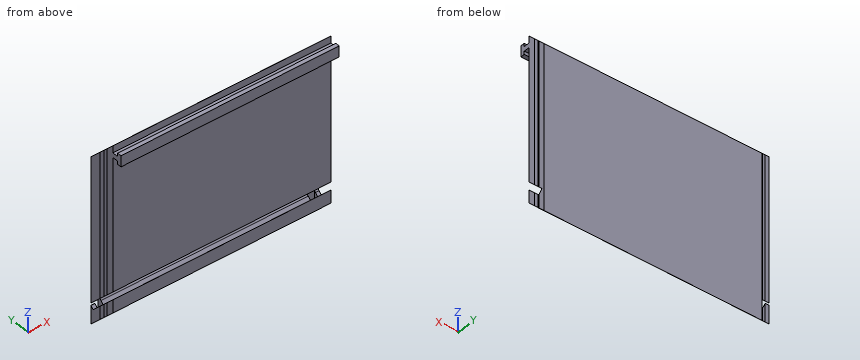
from build123d import *

# Parameters (mm, degrees)
SKETCH1_W           = 120
SKETCH1_H           = 100
BOSS_EXTRUDE1_DEPTH = 10
SKETCH2_W           = 6
SKETCH2_H           = 3
CUT_EXTRUDE1_DEPTH  = 120
SKETCH3_W           = 3
SKETCH3_H           = 1.75
CUT_EXTRUDE2_DEPTH  = 120
SKETCH4_W           = 3
SKETCH4_H           = 1.75
CUT_EXTRUDE3_DEPTH  = 120
SKETCH5_W           = 100
SKETCH5_H           = 3
BOSS_EXTRUDE2_DEPTH = 6
SKETCH6_W           = 3
SKETCH6_H           = 100
BOSS_EXTRUDE3_DEPTH = 1.75
SKETCH8_W           = 3
SKETCH8_H           = 100
BOSS_EXTRUDE4_DEPTH = 1.75
CUT_EXTRUDE4_DEPTH  = 140
CUT_EXTRUDE5_DEPTH  = 140
SKETCH12_W          = 120
SKETCH12_H          = 3
BOSS_EXTRUDE5_DEPTH = 6
SKETCH13_W          = 120
SKETCH13_H          = 3
BOSS_EXTRUDE6_DEPTH = 1.75
SKETCH14_W          = 120
SKETCH14_H          = 3
BOSS_EXTRUDE7_DEPTH = 1.75
SKETCH15_W          = 3.971349668
SKETCH15_H          = 100.27962334
CUT_EXTRUDE7_DEPTH  = 0.25
SKETCH16_W          = 3.977727367
SKETCH16_H          = 100.113606744
CUT_EXTRUDE8_DEPTH  = 0.25
SKETCH18_W          = 99.392543401
SKETCH18_H          = 7.459446395
CUT_EXTRUDE9_DEPTH  = 0.25
SKETCH19_W          = 3
SKETCH19_H          = 91.258373497
CUT_EXTRUDE10_DEPTH = 0.25
SKETCH22_W          = 3
SKETCH22_H          = 105.56058455
CUT_EXTRUDE11_DEPTH = 0.25
SKETCH23_W          = 145.417072626
SKETCH23_H          = 16.376201687
CUT_EXTRUDE12_DEPTH = 0.25
SKETCH24_W          = 92.054908244
SKETCH24_H          = 1.75
CUT_EXTRUDE13_DEPTH = 0.25
SKETCH25_W          = 91.75
SKETCH25_H          = 1.75
CUT_EXTRUDE14_DEPTH = 0.25
SKETCH27_W          = 146.123968395
SKETCH27_H          = 10.969132505
CUT_EXTRUDE15_DEPTH = 0.25
SKETCH28_W          = 131.910387722
SKETCH28_H          = 9.70209764
CUT_EXTRUDE16_DEPTH = 0.25
SKETCH29_W          = 147.06215687
SKETCH29_H          = 25.738379838
CUT_EXTRUDE17_DEPTH = 0.25
SKETCH30_W          = 120
SKETCH30_H          = 3
CUT_EXTRUDE18_DEPTH = 0.25
SKETCH31_W          = 120
SKETCH31_H          = 3
CUT_EXTRUDE19_DEPTH = 0.25
SKETCH32_W          = 120
SKETCH32_H          = 1.75
CUT_EXTRUDE20_DEPTH = 0.25
SKETCH33_W          = 120
SKETCH33_H          = 1.75
CUT_EXTRUDE21_DEPTH = 0.25
SKETCH36_W          = 96.5
SKETCH36_H          = 6.5
CUT_EXTRUDE23_DEPTH = 0.5
SKETCH39_W          = 96.5
SKETCH39_H          = 6.5
CUT_EXTRUDE27_DEPTH = 0.5
SKETCH41_W          = 4
SKETCH41_H          = 91.70363903
CUT_EXTRUDE28_DEPTH = 0.3
SKETCH42_W          = 3.987472746
SKETCH42_H          = 92.170181705
CUT_EXTRUDE29_DEPTH = 0.3
CUT_EXTRUDE30_DEPTH = 150
SKETCH44_W          = 120
SKETCH44_H          = 6
CUT_EXTRUDE31_DEPTH = 0.25
CUT_EXTRUDE32_DEPTH = 150


with BuildPart() as part:
    # Sketch1 → Boss-Extrude1 (new body)
    with BuildSketch(Plane(origin=(0, 0, 0), x_dir=(1, 0, 0), z_dir=(0, 1, 0))):
        with Locations((-60, -57.341499956)):
            Rectangle(SKETCH1_W, SKETCH1_H)
    extrude(amount=BOSS_EXTRUDE1_DEPTH)

    # Sketch2 → Cut-Extrude1 (cut)
    with BuildSketch(Plane(origin=(0, 0, 7.341499956), x_dir=(-1, 0, 0), z_dir=(0, 0, -1))):
        with Locations((3, 5)):
            Rectangle(SKETCH2_W, SKETCH2_H)
    extrude(amount=-CUT_EXTRUDE1_DEPTH, mode=Mode.SUBTRACT)

    # Sketch3 → Cut-Extrude2 (cut)
    with BuildSketch(Plane(origin=(0, 0, 7.341499956), x_dir=(-1, 0, 0), z_dir=(0, 0, -1))):
        with Locations((4.5, 7.375)):
            Rectangle(SKETCH3_W, SKETCH3_H)
    extrude(amount=-CUT_EXTRUDE2_DEPTH, mode=Mode.SUBTRACT)

    # Sketch4 → Cut-Extrude3 (cut)
    with BuildSketch(Plane(origin=(0, 0, 7.341499956), x_dir=(-1, 0, 0), z_dir=(0, 0, -1))):
        with Locations((4.5, 2.625)):
            Rectangle(SKETCH4_W, SKETCH4_H)
    extrude(amount=-CUT_EXTRUDE3_DEPTH, mode=Mode.SUBTRACT)

    # Sketch5 → Boss-Extrude2 (add)
    with BuildSketch(Plane.ZY.offset(120)):
        with Locations((57.341499956, 5)):
            Rectangle(SKETCH5_W, SKETCH5_H)
    extrude(amount=BOSS_EXTRUDE2_DEPTH)

    # Sketch6 → Boss-Extrude3 (add)
    with BuildSketch(Plane(origin=(0, 3.5, 0), x_dir=(-1, 0, 0), z_dir=(0, -1, 0))):
        with Locations((124.5, -57.341499956)):
            Rectangle(SKETCH6_W, SKETCH6_H)
    extrude(amount=BOSS_EXTRUDE3_DEPTH)

    # Sketch8 → Boss-Extrude4 (add)
    with BuildSketch(Plane(origin=(0, 6.5, 0), x_dir=(1, 0, 0), z_dir=(0, 1, 0))):
        with Locations((-124.5, -57.341499956)):
            Rectangle(SKETCH8_W, SKETCH8_H)
    extrude(amount=BOSS_EXTRUDE4_DEPTH)

    # Sketch9 → Cut-Extrude4 (cut)
    with BuildSketch(Plane(origin=(0, 0, 0), x_dir=(0, 0, -1), z_dir=(1, 0, 0))):
        Polygon((-7.341499956, 0), (-7.341499956, 10), (-17.341499956, 0), align=None)
    extrude(amount=-CUT_EXTRUDE4_DEPTH, mode=Mode.SUBTRACT)

    # Sketch10 → Cut-Extrude5 (cut)
    with BuildSketch(Plane(origin=(0, 0, 0), x_dir=(0, 0, -1), z_dir=(1, 0, 0))):
        Polygon((-107.341499956, 10), (-107.341499956, 0), (-97.341499956, 10), align=None)
    extrude(amount=-CUT_EXTRUDE5_DEPTH, mode=Mode.SUBTRACT)

    # Sketch12 → Boss-Extrude5 (add)
    with BuildSketch(Plane(origin=(0, 0, 0), x_dir=(-1, 0, 0), z_dir=(0, -1, 0))):
        with Locations((60, -102.341499956)):
            Rectangle(SKETCH12_W, SKETCH12_H)
    extrude(amount=BOSS_EXTRUDE5_DEPTH)

    # Sketch13 → Boss-Extrude6 (add)
    with BuildSketch(Plane(origin=(0, 0, 100.841499956), x_dir=(-1, 0, 0), z_dir=(0, 0, -1))):
        with Locations((60, -4.5)):
            Rectangle(SKETCH13_W, SKETCH13_H)
    extrude(amount=BOSS_EXTRUDE6_DEPTH)

    # Sketch14 → Boss-Extrude7 (add)
    with BuildSketch(Plane.XY.offset(103.841499956)):
        with Locations((-60, -4.5)):
            Rectangle(SKETCH14_W, SKETCH14_H)
    extrude(amount=BOSS_EXTRUDE7_DEPTH)

    # Sketch15 → Cut-Extrude7 (cut)
    with BuildSketch(Plane(origin=(0, 1.75, 0), x_dir=(-1, 0, 0), z_dir=(0, -1, 0))):
        with Locations((124.014325166, -55.451688286)):
            Rectangle(SKETCH15_W, SKETCH15_H)
    extrude(amount=-CUT_EXTRUDE7_DEPTH, mode=Mode.SUBTRACT)

    # Sketch16 → Cut-Extrude8 (cut)
    with BuildSketch(Plane(origin=(0, 8.25, 0), x_dir=(1, 0, 0), z_dir=(0, 1, 0))):
        with Locations((-124.011136317, -59.148303328)):
            Rectangle(SKETCH16_W, SKETCH16_H)
    extrude(amount=-CUT_EXTRUDE8_DEPTH, mode=Mode.SUBTRACT)

    # Sketch18 → Cut-Extrude9 (cut)
    with BuildSketch(Plane.ZY.offset(126)):
        with Locations((55.645228256, 5.729723198)):
            Rectangle(SKETCH18_W, SKETCH18_H)
    extrude(amount=-CUT_EXTRUDE9_DEPTH, mode=Mode.SUBTRACT)

    # Sketch19 → Cut-Extrude10 (cut)
    with BuildSketch(Plane(origin=(0, 6.5, 0), x_dir=(1, 0, 0), z_dir=(0, 1, 0))):
        with Locations((-121.5, -56.470686704)):
            Rectangle(SKETCH19_W, SKETCH19_H)
    extrude(amount=-CUT_EXTRUDE10_DEPTH, mode=Mode.SUBTRACT)

    # Sketch22 → Cut-Extrude11 (cut)
    with BuildSketch(Plane(origin=(0, 3.5, 0), x_dir=(-1, 0, 0), z_dir=(0, -1, 0))):
        with Locations((121.5, -51.061207681)):
            Rectangle(SKETCH22_W, SKETCH22_H)
    extrude(amount=-CUT_EXTRUDE11_DEPTH, mode=Mode.SUBTRACT)

    # Sketch23 → Cut-Extrude12 (cut)
    with BuildSketch(Plane.ZY.offset(125.75)):
        with Locations((82.050036269, -0.188100844)):
            Rectangle(SKETCH23_W, SKETCH23_H)
    extrude(amount=-CUT_EXTRUDE12_DEPTH, mode=Mode.SUBTRACT)

    # Sketch24 → Cut-Extrude13 (cut)
    with BuildSketch(Plane(origin=(-123, 0, 0), x_dir=(0, 0, -1), z_dir=(1, 0, 0))):
        with Locations((-59.314045834, 2.875)):
            Rectangle(SKETCH24_W, SKETCH24_H)
    extrude(amount=-CUT_EXTRUDE13_DEPTH, mode=Mode.SUBTRACT)

    # Sketch25 → Cut-Extrude14 (cut)
    with BuildSketch(Plane(origin=(-123, 0, 0), x_dir=(0, 0, -1), z_dir=(1, 0, 0))):
        with Locations((-55.216499956, 7.125)):
            Rectangle(SKETCH25_W, SKETCH25_H)
    extrude(amount=-CUT_EXTRUDE14_DEPTH, mode=Mode.SUBTRACT)

    # Sketch27 → Cut-Extrude15 (cut)
    with BuildSketch(Plane(origin=(0, -6, 0), x_dir=(-1, 0, 0), z_dir=(0, -1, 0))):
        with Locations((46.938015803, -100.106933704)):
            Rectangle(SKETCH27_W, SKETCH27_H)
    extrude(amount=-CUT_EXTRUDE15_DEPTH, mode=Mode.SUBTRACT)

    # Sketch28 → Cut-Extrude16 (cut)
    with BuildSketch(Plane.XY.offset(105.591499956)):
        with Locations((-65.955193861, -7.85104882)):
            Rectangle(SKETCH28_W, SKETCH28_H)
    extrude(amount=-CUT_EXTRUDE16_DEPTH, mode=Mode.SUBTRACT)

    # Sketch29 → Cut-Extrude17 (cut)
    with BuildSketch(Plane(origin=(0, 0, 99.091499956), x_dir=(-1, 0, 0), z_dir=(0, 0, -1))):
        with Locations((46.468921565, -15.869189919)):
            Rectangle(SKETCH29_W, SKETCH29_H)
    extrude(amount=-CUT_EXTRUDE17_DEPTH, mode=Mode.SUBTRACT)

    # Sketch30 → Cut-Extrude18 (cut)
    with BuildSketch(Plane(origin=(0, 0, 100.841499956), x_dir=(-1, 0, 0), z_dir=(0, 0, -1))):
        with Locations((60, -1.5)):
            Rectangle(SKETCH30_W, SKETCH30_H)
    extrude(amount=-CUT_EXTRUDE18_DEPTH, mode=Mode.SUBTRACT)

    # Sketch31 → Cut-Extrude19 (cut)
    with BuildSketch(Plane.XY.offset(103.841499956)):
        with Locations((-60, -1.5)):
            Rectangle(SKETCH31_W, SKETCH31_H)
    extrude(amount=-CUT_EXTRUDE19_DEPTH, mode=Mode.SUBTRACT)

    # Sketch32 → Cut-Extrude20 (cut)
    with BuildSketch(Plane(origin=(0, -3, 0), x_dir=(1, 0, 0), z_dir=(0, 1, 0))):
        with Locations((-60, -104.466499956)):
            Rectangle(SKETCH32_W, SKETCH32_H)
    extrude(amount=-CUT_EXTRUDE20_DEPTH, mode=Mode.SUBTRACT)

    # Sketch33 → Cut-Extrude21 (cut)
    with BuildSketch(Plane(origin=(0, -3, 0), x_dir=(1, 0, 0), z_dir=(0, 1, 0))):
        with Locations((-60, -100.216499956)):
            Rectangle(SKETCH33_W, SKETCH33_H)
    extrude(amount=-CUT_EXTRUDE21_DEPTH, mode=Mode.SUBTRACT)

    # Sketch36 → Cut-Extrude23 (cut)
    with BuildSketch(Plane.ZY.offset(3)):
        with Locations((57.341499956, 5)):
            Rectangle(SKETCH36_W, SKETCH36_H)
    extrude(amount=-CUT_EXTRUDE23_DEPTH, mode=Mode.SUBTRACT)

    # Sketch39 → Cut-Extrude27 (cut)
    with BuildSketch(Plane.ZY.offset(2.5)):
        with Locations((57.341499956, 5)):
            Rectangle(SKETCH39_W, SKETCH39_H)
    extrude(amount=-CUT_EXTRUDE27_DEPTH, mode=Mode.SUBTRACT)

    # Sketch41 → Cut-Extrude28 (cut)
    with BuildSketch(Plane(origin=(0, 1.75, 0), x_dir=(1, 0, 0), z_dir=(0, 1, 0))):
        with Locations((-4, -61.443319471)):
            Rectangle(SKETCH41_W, SKETCH41_H)
    extrude(amount=-CUT_EXTRUDE28_DEPTH, mode=Mode.SUBTRACT)

    # Sketch42 → Cut-Extrude29 (cut)
    with BuildSketch(Plane(origin=(0, 8.25, 0), x_dir=(-1, 0, 0), z_dir=(0, -1, 0))):
        with Locations((3.993736373, -52.972884842)):
            Rectangle(SKETCH42_W, SKETCH42_H)
    extrude(amount=-CUT_EXTRUDE29_DEPTH, mode=Mode.SUBTRACT)

    # Sketch43 → Cut-Extrude30 (cut)
    with BuildSketch(Plane(origin=(0, 0, 0), x_dir=(0, 0, -1), z_dir=(1, 0, 0))):
        Polygon((-19.32678133, 7.914213562), (-33.468916954, -6.227922061), (-32.054703391, -7.642135624), (-17.912567767, 6.5), align=None)
    extrude(amount=-CUT_EXTRUDE30_DEPTH, mode=Mode.SUBTRACT)

    # Sketch44 → Cut-Extrude31 (cut)
    with BuildSketch(Plane(origin=(0, -5.75, 0), x_dir=(-1, 0, 0), z_dir=(0, -1, 0))):
        with Locations((60, -102.341499956)):
            Rectangle(SKETCH44_W, SKETCH44_H)
    extrude(amount=-CUT_EXTRUDE31_DEPTH, mode=Mode.SUBTRACT)

    # Sketch45 → Cut-Extrude32 (cut)
    with BuildSketch(Plane(origin=(0, 0, 0), x_dir=(0, 0, -1), z_dir=(1, 0, 0))):
        Polygon((-19.32678133, 7.914213562), (-20.033888111, 8.621320344), (-29.487832781, -0.832624327), (-28.780726, -1.539731108), align=None)
    extrude(amount=-CUT_EXTRUDE32_DEPTH, mode=Mode.SUBTRACT)


solid = part.part
Here's how the part is built. I have some questions about the finished solid (model axes, mm). Coordinates: 2 decimals unless noted, no trailing zeros. Write each loop counter-clockwise with the first axis right and the second up, starting at its lowest first coordinate (ties: lowest second). Pieces come first, ordered by that corner, then holes.
1) If we section it at B-B (x = -18.5): List the corners of the cut face in (y, z) for me.
Filled in:
outline: (-5.5, 99.34) - (-3.25, 99.34) - (-3.25, 101.09) - (0, 101.09) - (0, 28.66) - (8.62, 20.03) - (6.5, 17.91) - (0, 24.41) - (0, 17.34) - (10, 7.34) - (10, 97.34) - (0, 107.34) - (0, 103.59) - (-3.25, 103.59) - (-3.25, 105.34) - (-5.5, 105.34) - close
2) If we section it at C-C (y = -1.5): List the corners of the cut face in (x, z) for me, plus the area to 3 significant figures.
Filled in:
outline: (-120, 101.09) - (0, 101.09) - (0, 103.59) - (-120, 103.59) - close
area: 300 mm2
3) If I drill on line 1 (X direction, y = 7.5, z = 39); line 2 (Z direction, x = -54, y = 8); line 3 (X direction, y = 8.5, z = 50.5), over which ranges is the centre line in solid material (lowest first)?
Filled in:
line 1: x = -125.5 to -123.25, -120 to -6, -2 to 0
line 2: z = 9.34 to 19.41, 20.66 to 99.34
line 3: x = -120 to -5.99, -2 to 0
4) I'm going to push flat-ended pins straight in: pin 1 (1.4 mm diameter, centred on x = -67.5, z = 100.5, fed in from +Y); pin 2 (0.7 mm diameter, centred on x = -87, y = -4, fed in from -Z); pin 3 (3 mm diameter, centred on x = -112.5, z = 76.5, fed in from -Y). Where does each tip first touch, or does it pass through?
Filled in:
pin 1: stops at y = 7.54
pin 2: stops at z = 99.34
pin 3: stops at y = 0
